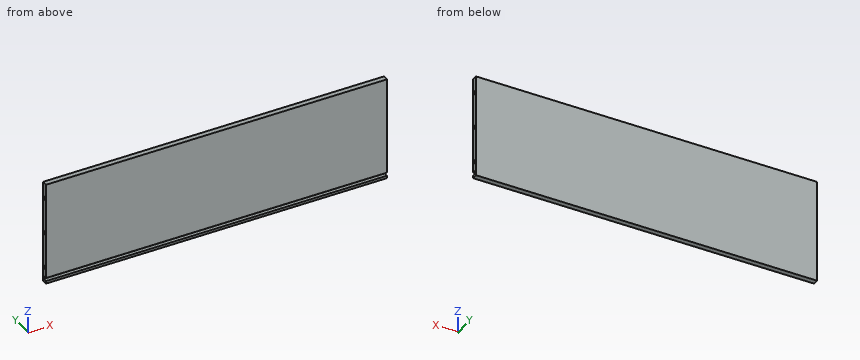
```python
from build123d import *

# Parameters (mm, degrees)
F0_W     = 823.976
F0_H     = 254
F1_DEPTH = 12.7
F2_W     = 823.976
F2_H     = 7.874
F3_DEPTH = 9.652
F5_D     = 8.001
F5_DEPTH = 25.4
F5_TIP   = 2.4037429064
F7_D     = 8.001
F7_DEPTH = 25.4
F7_TIP   = 2.4037429064


with BuildPart() as f1:
    # F0 (on Front) → F1 (new body)
    with BuildSketch(Plane.XZ):
        Rectangle(F0_W, F0_H)
    extrude(amount=F1_DEPTH)

    # F2 (on face) → F3 (cut)
    with BuildSketch(Plane.XZ.offset(12.7)):
        with Locations((0, -116.713)):
            Rectangle(F2_W, F2_H)
    extrude(amount=-F3_DEPTH, mode=Mode.SUBTRACT)

    # F5
    with Locations(Plane(origin=(-411.988, 0, 0), x_dir=(0, -1, 0), z_dir=(-1, 0, 0))):
        with Locations((6.35, 88.9), (6.35, 0), (6.35, -88.9)):
            Hole(F5_D / 2, depth=F5_DEPTH)
            with Locations((0, 0, -(F5_DEPTH + F5_TIP / 2))):  # 118° drill point
                Cone(0, F5_D / 2, F5_TIP, mode=Mode.SUBTRACT)

    # F7
    with Locations(Plane.YZ.offset(411.988)):
        with Locations((-6.35, 88.9), (-6.35, 0), (-6.35, -88.9)):
            Hole(F7_D / 2, depth=F7_DEPTH)
            with Locations((0, 0, -(F7_DEPTH + F7_TIP / 2))):  # 118° drill point
                Cone(0, F7_D / 2, F7_TIP, mode=Mode.SUBTRACT)


solid = f1.part
```
CAD build for the part. Positions are in the model's coordinates, mm. Coordinates: 2 decimals unless noted, no trailing zeros. Order: outer loops, then holes, each group sorted by start corner. A loop starts at its lowest first (then second) coordinate and runs counter-clockwise, first axis right, second up. Notation, with made-up numbers: (16.5, 48) - (35.5, 48) arc R19 cw to (35.5, 72) - close; hole circle Ø1 at (34, -0.5). An arc over 180 degrees is marked (long way). Use a Markdown table: item, result. Add a question column.
(1) Flat gauge pins, fed straight in: pin 1 (7 mm diameter, centred on y = -6.35, z = 88.9, fed in from -X); pin 2 (7 mm diameter, centred on y = -6.35, z = 0, fed in from +X); pin 3 (6.5 mm diameter, centred on y = -6.35, z = -88.9, fed in from -X). Where does each tip first touch, or does it go through?
(2) Saw through at A-A (x = -7.5). Give the cut face in (y, z), then the cut area to 3 significant figures.
(3) Drill centre lines: line 1 along Z through (x, y) = (392.75, -6.35); line 2 along Y through (x, z) = (398, 0); line 3 along Z through (x, y) = (-239.5, -6.5). Where is each one in solid material? Low to high. Write a range as [from, to].
Solved:
| question | item | result |
|---|---|---|
| 1 | pin 1 | stops at x = -386.29 |
| 1 | pin 2 | stops at x = 386.29 |
| 1 | pin 3 | stops at x = -386.14 |
| 2 | outline | (-12.7, -127) - (0, -127) - (0, 127) - (-12.7, 127) - (-12.7, -112.78) - (-3.05, -112.78) - (-3.05, -120.65) - (-12.7, -120.65) - close |
| 2 | area | 3,150 mm² |
| 3 | line 1 | z = [-127, -120.65], [-112.78, -92.9], [-84.9, -4], [4, 84.9], [92.9, 127] |
| 3 | line 2 | y = [-12.7, -10.35], [-2.35, 0] |
| 3 | line 3 | z = [-127, -120.65], [-112.78, 127] |
